Geometry check sheet. Reference: the model listing, model coordinates, mm. Give positions to 0.01 mm unless a question says otherwise; leave off trailing zeros. Loops run counter-clockwise (first coordinate to the right, second up) from the corner with the lowest first, then second, coordinate; pieces in that order, holes last. Notation, with made-up numbers: (37.25, 26.5) -> (79.25, 26.5) arc R18 cw to (79.25, 60.5) -> close; hole circle Ø10 at (64, 66.25). An arc over 180 degrees is marked (long way). Answer in a Markdown table with one row per item. Add a question column.
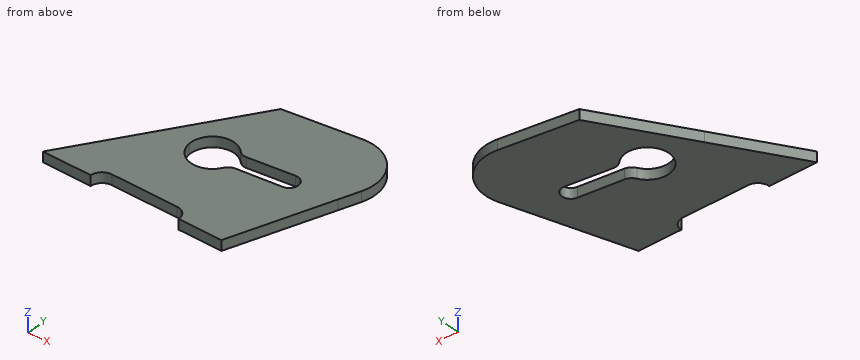
```python
from build123d import *

# Parameters (mm, degrees)
BOSS_EXTRUDE1_DEPTH = 8


with BuildPart() as part:
    # Sketch2 → Boss-Extrude1 (new body)
    with BuildSketch(Plane.XY):
        with BuildLine():
            Line((79.487889635, 127.207214423), (37.624267761, 60.211414827))
            Line((37.624267761, 60.211414827), (61.402056741, 63.469750476))
            ThreePointArc((61.402056741, 63.469750476), (70.67132686, 80.997615577), (90.243088989, 77.820895466))
            ThreePointArc((90.243088989, 77.820895466), (93.32868479, 75.909168155), (96.941453957, 75.557740071))
            Line((96.941453957, 75.557740071), (131.814885044, 80.183965492))
            ThreePointArc((131.814885044, 80.183965492), (136.979315131, 78.811568483), (139.670612135, 74.195105322))
            Line((139.670612135, 74.195105322), (167.339393539, 77.986634336))
            Line((167.339393539, 77.986634336), (172.50354814, 93.880267937))
            ThreePointArc((172.50354814, 93.880267937), (166.569139078, 124.354715336), (137.573015724, 135.451290736))
            Line((137.573015724, 135.451290736), (79.487889635, 127.207214423))
        make_face()
        with BuildLine():
            Line((37.624267761, 60.211414827), (0, 0))
            Line((0, 0), (38, 0))
            ThreePointArc((38, 0), (40.636038969, 6.363961031), (47, 9))
            Line((47, 9), (99, 9))
            ThreePointArc((99, 9), (105.363961031, 6.363961031), (108, 0))
            Line((108, 0), (142, 0))
            Line((142, 0), (167.339393539, 77.986634336))
            Line((167.339393539, 77.986634336), (139.670612135, 74.195105322))
            ThreePointArc((139.670612135, 74.195105322), (138.274512361, 68.964746138), (133.565613448, 66.29416141))
            Line((133.565613448, 66.29416141), (99.495664198, 62.224794823))
            ThreePointArc((99.495664198, 62.224794823), (95.888310918, 60.857089082), (93.340518027, 57.960130667))
            ThreePointArc((93.340518027, 57.960130667), (75.354717379, 49.025178799), (61.402056741, 63.469750476))
            Line((61.402056741, 63.469750476), (37.624267761, 60.211414827))
        make_face()
    extrude(amount=BOSS_EXTRUDE1_DEPTH)


solid = part.part
```
1. Sectioned sample at A-A (z = 6.75). Enter the section's corners in (x, y), plus the area to 3 significant figures.
2. Sectioned sample at D-D (y = 121). Enter the section's corners in (x, z), plus the area to 3 significant figures.
3. Material ranges on L1, parallel to Y at x = 128.5, z = 1.5; L2, parallel to Y at x = 103.5, z = 2; L3, parallel to X at y = 73.5, z = 2.5, recorded low to high. Write a range as from..to.
4. Gauge pin test, flat ends, axial feed: pin 1 Ø4 at (y, z) = (59.5, 3.5) entering from -X; pin 2 Ø4 at (x, z) = (83.5, 2.5) entering from -Y. Record the tip position at first contact, or that the pin passes through.
5. Sectioned sample at B-B (x = 113.5). Enter the section's corners in (y, z), plus the area to 3 significant figures.
6. Sectioned sample at C-C (x = 77.5). Enter the section's corners in (y, z), plus the area to 3 significant figures.
Response:
| question | item | result |
|---|---|---|
| 1 | outline | (0, 0) -> (38, 0) arc R9 cw to (47, 9) -> (99, 9) arc R9 cw to (108, 0) -> (142, 0) -> (172.5, 93.88) arc R32 ccw to (137.57, 135.45) -> (79.49, 127.21) -> close; hole (90.24, 77.82) arc R17 ccw (long way) to (93.34, 57.96) arc R8 cw to (99.5, 62.22) -> (133.57, 66.29) arc R7 ccw (long way) to (131.81, 80.18) -> (96.94, 75.56) arc R8 cw to start |
| 1 | area | 13,700 mm2 |
| 2 | outline | (75.61, 0) -> (169.03, 0) -> (169.03, 8) -> (75.61, 8) -> close |
| 2 | area | 747 mm2 |
| 3 | L1 | y = 0..65.69, 79.74..134.16 |
| 3 | L2 | y = 7.79..62.7, 76.43..130.62 |
| 3 | L3 | x = 45.93..63.1, 139.73..165.88 |
| 4 | pin 1 | stops at x = 35.93 |
| 4 | pin 2 | stops at y = 9 |
| 5 | outline | (0, 0) -> (63.9, 0) -> (63.9, 8) -> (0, 8) -> close; (77.75, 0) -> (132.03, 0) -> (132.03, 8) -> (77.75, 8) -> close |
| 5 | area | 945 mm2 |
| 6 | outline | (9, 0) -> (48.79, 0) -> (48.79, 8) -> (9, 8) -> close; (82.76, 0) -> (124.03, 0) -> (124.03, 8) -> (82.76, 8) -> close |
| 6 | area | 648 mm2 |
